```python
from build123d import *

# Parameters (mm, degrees)
SKETCH1_R           = 14.75
BOSS_EXTRUDE1_DEPTH = 18
SKETCH2_R           = 23.1
BOSS_EXTRUDE2_DEPTH = 10
SKETCH3_R           = 26
BOSS_EXTRUDE3_DEPTH = 74
SKETCH4_R           = 26
SKETCH4_R_2         = 25.5
CUT_EXTRUDE1_DEPTH  = 18


with BuildPart() as part:
    # Sketch1 → Boss-Extrude1 (new body)
    with BuildSketch(Plane(origin=(0, 0, 0), x_dir=(1, 0, 0), z_dir=(0, 1, 0))):
        Circle(SKETCH1_R)
    extrude(amount=BOSS_EXTRUDE1_DEPTH)

    # Sketch2 → Boss-Extrude2 (add)
    with BuildSketch(Plane(origin=(0, 18, 0), x_dir=(1, 0, 0), z_dir=(0, 1, 0))):
        Circle(SKETCH2_R)
    extrude(amount=BOSS_EXTRUDE2_DEPTH)

    # Sketch3 → Boss-Extrude3 (add)
    with BuildSketch(Plane(origin=(0, 28, 0), x_dir=(1, 0, 0), z_dir=(0, 1, 0))):
        Circle(SKETCH3_R)
    extrude(amount=BOSS_EXTRUDE3_DEPTH)

    # Sketch4 → Cut-Extrude1 (cut)
    with BuildSketch(Plane(origin=(0, 102, 0), x_dir=(1, 0, 0), z_dir=(0, 1, 0))):
        Circle(SKETCH4_R)
        Circle(SKETCH4_R_2, mode=Mode.SUBTRACT)
    extrude(amount=-CUT_EXTRUDE1_DEPTH, mode=Mode.SUBTRACT)


solid = part.part
```
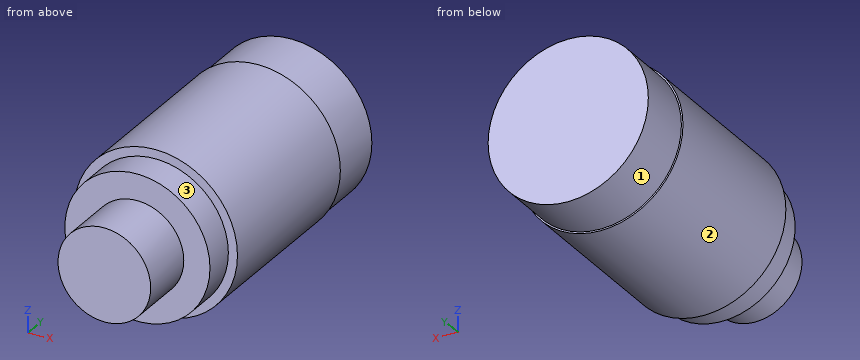
Design review of the part built by this model. Coordinates are the model's own, in mm. Face numbers are marked on the shaded views. A direction names the side the tool comes from. Give positions to 0.01 mm unless a question says otherwise; leave off trailing zeros. Write each loop counter-clockwise with the first axis right and the second up, starting at its lowest first coordinate (ties: lowest second). Pieces come first, ordered by that corner, then holes.
(1) Add section C-C (y = 64.5). Give the boundary of the cut face in (x, z), and give its area (3 significant figures).
Checked values:
outline: circle Ø52 at (0, 0)
area: 2,120 mm2
(2) Add section D-D (x = 20). Give the boundary of the cut face in (y, z), and give its area (3 significant figures).
Checked values:
outline: (18, -11.56) - (28, -11.56) - (28, -16.61) - (84, -16.61) - (84, -15.82) - (102, -15.82) - (102, 15.82) - (84, 15.82) - (84, 16.61) - (28, 16.61) - (28, 11.56) - (18, 11.56) - close
area: 2,660 mm2
(3) Add section A-A (x = 0). Give the boundary of the cut face in (y, z).
Checked values:
outline: (0, -14.75) - (18, -14.75) - (18, -23.1) - (28, -23.1) - (28, -26) - (84, -26) - (84, -25.5) - (102, -25.5) - (102, 25.5) - (84, 25.5) - (84, 26) - (28, 26) - (28, 23.1) - (18, 23.1) - (18, 14.75) - (0, 14.75) - close
(4) Clearance check with flat-ended pins moving along their axes: pin 1 Ø12 at (x, y) = (-10.5, 83.5) entering from -Z; pin 2 Ø5 at (x, y) = (-1, 37) entering from -Z; pin 3 Ø6 at (x, y) = (12, 69.5) entering from +Z. State where each tip first meets the part, or that it passes through.
Checked values:
pin 1: stops at z = -25.61
pin 2: stops at z = -26
pin 3: stops at z = 24.39
(5) Add section B-B (z = 0). Give the boundary of the cut face in (x, y), and give its area (3 significant figures).
Checked values:
outline: (-26, 28) - (-23.1, 28) - (-23.1, 18) - (-14.75, 18) - (-14.75, 0) - (14.75, 0) - (14.75, 18) - (23.1, 18) - (23.1, 28) - (26, 28) - (26, 84) - (25.5, 84) - (25.5, 102) - (-25.5, 102) - (-25.5, 84) - (-26, 84) - close
area: 4,820 mm2
(6) Tool access review of the marked faces 1, 2 and 3: name each direction out of +Z, -Z, +X, -X, +Y, -Y from which nothing blocks a thin tool from reaching the whole face with its end or side.
Checked values:
face 1: +Y
face 2: +Y, -Y
face 3: -Y
(7) Wall thickness on line 1 along X through (y, z) = (92.5, 0.5); line 2 along Y through (x, z) = (19, 14); line 3 along Y through (x, z) = (-15.5, 3): over which ranges is each line inside the solid? List them lowest first.
Checked values:
line 1: x = -25.5 to 25.5
line 2: y = 28 to 102
line 3: y = 18 to 102
